from build123d import *

# Parameters (mm, degrees)
F0_W     = 150
F0_H     = 140
F1_DEPTH = 86
F2_R     = 1.5
F3_DEPTH = 10
F4_R     = 60
F5_DEPTH = 3


with BuildPart() as f1:
    # F0 (on Top) → F1 (new body)
    with BuildSketch(Plane.XY):
        with Locations((75, 70)):
            Rectangle(F0_W, F0_H)
    extrude(amount=F1_DEPTH)

    # F2 (on face) → F3 (cut)
    with BuildSketch(Plane.XZ):
        with Locations((6, 80)):
            Circle(F2_R)
        with Locations((6, 16)):
            Circle(F2_R)
        with Locations((144, 80)):
            Circle(F2_R)
        with Locations((120, 6)):
            Circle(F2_R)
    extrude(amount=-F3_DEPTH, mode=Mode.SUBTRACT)

    # F4 (on face) → F5 (cut)
    with BuildSketch(Plane.XY.offset(86)):
        with Locations((65, 70)):
            Circle(F4_R)
    extrude(amount=-F5_DEPTH, mode=Mode.SUBTRACT)


solid = f1.part
Model file for the job. Use its own axes, mm. A direction names the side the tool comes from. Round coordinates to 2 decimals unless told otherwise and drop trailing zeros. Loops run counter-clockwise (first coordinate to the right, second up) from the corner with the lowest first, then second, coordinate; pieces in that order, holes last. Notation, with made-up numbers: (31.5, -3) - (51.5, -3) arc R30 cw to (51.5, 27) - close; hole circle Ø2 at (-1, 25). An arc over 180 degrees is marked (long way). Write each question's results on one line, items separated by ' | '.
(1) Mould opens along X. For faces 3 (the flat face through (64, 71, 83)), 4 (the flat face through (124, 87, 86)), 5 (the flat face through (0, 69, 42)) say: released by +X, released by -X, zero draft, split by the parting line, or undercut.
Answer below:
face 3: undercut | face 4: zero draft | face 5: released by -X
(2) Saw through at A-A, the plane x = 29. List the corners of the cut face in (y, z), then the cut area to 3 significant figures.
Answer below:
outline: (0, 0) - (140, 0) - (140, 86) - (118, 86) - (118, 83) - (22, 83) - (22, 86) - (0, 86) - close | area: 11,800 mm^2
(3) Saw through at B-B, the plane y = 70. List the corners of the cut face in (x, z), then the cut area to 3 significant figures.
Answer below:
outline: (0, 0) - (150, 0) - (150, 86) - (125, 86) - (125, 83) - (5, 83) - (5, 86) - (0, 86) - close | area: 12,500 mm^2
(4) 3-axis set-ups, long thin cutter, end or side, ignore diameter. For faces 1 (the flat face through (74, 140, 42)), 2 (the cylindrical face through (17.386, 33.491, 84.521)): which of +Z, -Z, +X, -X, +Y, -Y reach the whole face in a straight line?
Answer below:
face 1: +Z, -Z, +X, -X, +Y | face 2: +Z
(5) Wall check: L1, parallel to Z at x = 6, y = 5; L2, parallel to Y at x = 65, z = 84; L3, parallel to Z at x = 120, y = 4. Give the ranges that are in metal, low to high.
Answer below:
L1: z = 0 to 14.5, 17.5 to 78.5, 81.5 to 86 | L2: y = 0 to 10, 130 to 140 | L3: z = 0 to 4.5, 7.5 to 86
(6) Pin check, flat tips, straight feed: pin 1 (2.5 mm diameter, centred on x = 143.5, z = 80.5, fed in from -Y); pin 2 (2 mm diameter, centred on x = 93.5, y = 36, fed in from +Z); pin 3 (2.5 mm diameter, centred on x = 144, z = 80, fed in from -Y). Stop position of each tip, or through.
Answer below:
pin 1: stops at y = 0 | pin 2: stops at z = 83 | pin 3: stops at y = 10
